Autodesk Inventor part; units mm, degrees
ref_plane "Work Plane1" through (-3, 0, -45) normal (-0.9469, 0, -0.3214) x (0, -1, 0)
ref_plane "Work Plane2" through (-3, 0, 0) normal (-0.9469, 0, 0.3214) x (0, -1, 0)
ref_plane "YZ Plane" through (0, 0, 0) normal (1, 0, 0) x (0, 1, 0)
sketch "Sketch1" plane through (0, 0, 0) normal (0, 1, 0) x (-1, 0, 0)
  line L0 (0, 0) -> (0, -45) construction
  arc A0 (0, -45) -> (0, 0) centre (-66.2854, -22.5) ccw
  line L1 (0, 0) -> (3, 0)
  line L2 (0, -45) -> (3, -45)
  arc A1 (3, -45) -> (3, 0) centre (-63.2854, -22.5) ccw
  dimension "d0" = 45
  dimension "d1" = 70
  dimension "d2" = 3
  dimension "d3" = 3
  dimension "d4" = 70
extrude "Extrusion1" add sketch "Sketch1" along normal blind 40
ref_plane "Work Plane1" through (-3, 0, -45) normal (-0.9469, 0, -0.3214) x (0, -1, 0)
sketch "Sketch2" plane through (-3, 0, -45) normal (-0.9469, 0, -0.3214) x (0, -1, 0)
  line L0 (-40, 42.612) -> (-40, 0)
  line L1 (0, -0.9643) -> (-40, -0.9643)
  point P0 (0, 41.6477)
  point P1 (-30, 9.0357)
  dimension "d7" = 10
  dimension "d8" = 10
hole "Hole1" at (-5.9043, 30, -36.4438) direction (0.9469, 0, 0.3214) diameter 3.5 end through all
ref_plane "Work Plane2" through (-3, 0, 0) normal (-0.9469, 0, 0.3214) x (0, -1, 0)
sketch "Sketch3" plane through (-3, 0, 0) normal (-0.9469, 0, 0.3214) x (0, -1, 0)
  line L0 (0, 0.9643) -> (-40, 0.9643)
  line L1 (-40, 0) -> (-40, -42.612)
  point P0 (-30, -9.0357)
  dimension "d16" = 10
  dimension "d17" = 10
hole "Hole2" at (-5.9043, 30, -8.5562) direction (0.9469, 0, -0.3214) diameter 3.5 end through all
sketch "Sketch4" plane through (0, 0, 0) normal (1, 0, 0) x (0, 1, 0)
  line L0 (0, -45) -> (40, -45)
  line L1 (0, 0) -> (40, 0)
  line L2 (0, -45) -> (0, 0)
  line L3 (0, 0) -> (40, 0)
  line L4 (40, -45) -> (40, 0)
  line L5 (0, -45) -> (40, -45)
  line L6 (0, 0) -> (0, -22)
  line L7 (20, -45) -> (10.7074, -22)
  line L8 (10.7074, -22) -> (0, -22)
  line L9 (20, -45) -> (0, -45)
  line L10 (0, -22) -> (0, -45)
  point P0 (30, -7.0213)
  point P1 (30, -34.518)
  point P2 (20, 0)
  dimension "d25" = 22
  dimension "d26" = 112
extrude "Extrusion2" cut sketch "Sketch4" against normal up to next contours L2 L8 L7 L0
properties part number "cap_mount"
CAD build for the part. Positions are in the model's coordinates, mm. A direction names the side the tool comes from. Round coordinates to 2 decimals unless told otherwise and drop trailing zeros. Order: outer loops, then holes, each group sorted by start corner. A loop starts at its lowest first (then second) coordinate and runs counter-clockwise, first axis right, second up. Notation, with made-up numbers: M -3.5,-38 L 44.5,-38 A13 ccw 44.5,-13 Z; hole C 46,37 d7. An arc over 180 degrees is marked long. Use one line per item in the form item = value.
Q1. Saw through at C-C on y = 9. Give the cut face in (x, z), then the cut area to 3 significant figures.
Recorded:
outline = M -6.71,-22 L -3.71,-22 A70 cw 0,0 L -3,0 A70 ccw Z
area = 66.0 mm^2
Q2. Saw through at A-A on x = -1.5. Give the cut face in (y, z), then the cut area to 3 significant figures.
Recorded:
outline = M 0,-5.03 L 40,-5.03 L 40,0 L 0,0 Z; M 17.97,-39.97 L 20,-45 L 40,-45 L 40,-39.97 Z
area = 307 mm^2
Q3. Saw through at D-D on x = -4.25. State how many separate pieces and enclosed holes the cut face has, then the cut area to 3 significant figures.
Recorded:
separate_pieces = 1
enclosed_holes = 2
area = 1,180 mm^2
Q4. Probe L1, parallel to Y at x = -3.25, z = -37; L2, parallel to Y at x = -3, z = -36; L3, parallel to X at y = 28, z = -17.5. List the from-to ranges inside material, lowest first.
Recorded:
L1 = 16.77 to 28.92, 31.08 to 40
L2 = 16.36 to 28.33, 31.67 to 40
L3 = -6.54 to -3.54
Q5. Which spindle directions (+Z, -Z, +X, -X, +Y, -Y) get a long thin tool onto all of the face, cutting with end or side? Do faces 1 (the cylindrical face through (-4.189, 28.524, -34.868)), 2 (the flat face through (-5, 5, -22)). Say none if no direction does.
Recorded:
face_1 = none
face_2 = -Z, +X, -X, -Y
Q6. Flat gauge pins, fed straight in: P1, Ø5, axis at y = 30, z = -15.5, coming from the +X side; P2, Ø0.9, axis at x = -6, y = 3.5, coming from the -Z side; P3, Ø5, axis at y = 11.5, z = -9.5, coming from the +X side. Where does each tip first touch, or does it go through?
Recorded:
P1 = -3.07
P2 = -22
P3 = -1.98
Q7. Two-plate mould, pull along Y, no slides. Class faces 3 (the cylindrical face through (-3.35, 29.47, -7.66)), 4 (the flat face through (-4, 40, -22)), 5 (the flat face through (-1, 30, -45)): +Y half, -Y half, draft (parallel to the pull), parting line (faces both ways), or undercut.
Recorded:
face_3 = undercut
face_4 = +Y half
face_5 = draft
Q8. Saw through at B-B on z = -26. Give the cut face in (x, y), then the cut area to 3 significant figures.
Recorded:
outline = M -6.63,12.32 L -3.63,12.32 L -3.63,40 L -6.63,40 Z
area = 83.0 mm^2
